```python
from build123d import *

# Parameters (mm, degrees)
RESSALTO_EXTRUS_O1_DEPTH                             = 4
FURO_DE_DI_METRO_6_0_6_1_D                           = 6
FURO_DE_DI_METRO_6_0_6_1_DEPTH                       = 2
FURO_DE_DI_METRO_6_0_6_1_TIP                         = 1.802581857
ESBO_O4_R                                            = 1.2
CORTE_EXTRUS_O1_DEPTH                                = 32.271167096
ESCAREADO_PARA_PARAFUSO_COM_CABE_A_ESCAR_D           = 3.4
ESCAREADO_PARA_PARAFUSO_COM_CABE_A_ESCAR_CSINK_D     = 6.3
ESCAREADO_PARA_PARAFUSO_COM_CABE_A_ESCAR_CSINK_ANGLE = 90
FILETE1_R                                            = 10
FILETE2_R                                            = 1


with BuildPart() as part:
    # Esboço1 → Ressalto-extrusão1 (new body)
    with BuildSketch(Plane(origin=(0, 0, 0), x_dir=(0, 0, -1), z_dir=(1, 0, 0))):
        with BuildLine():
            Line((0, 0), (0, 3.091839499))
            ThreePointArc((0, 3.091839499), (2.870368785, 6.92901728), (7.361966659, 5.259137398))
            Line((7.361966659, 5.259137398), (16.225984495, -7.134144996))
            Line((16.225984495, -7.134144996), (26, -16.908160501))
            Line((26, -16.908160501), (13, -16.908160501))
            Line((13, -16.908160501), (8, -11.908160501))
            Line((8, -11.908160501), (8, -8.399335203))
            Line((8, -8.399335203), (0, 0))
        make_face()
    extrude(amount=RESSALTO_EXTRUS_O1_DEPTH)

    # Furo de diâmetro Ø6.0 (6)1
    with Locations(Plane.ZY):
        with Locations((-4, 3.091839499)):
            Hole(FURO_DE_DI_METRO_6_0_6_1_D / 2, depth=FURO_DE_DI_METRO_6_0_6_1_DEPTH)
            with Locations((0, 0, -(FURO_DE_DI_METRO_6_0_6_1_DEPTH + FURO_DE_DI_METRO_6_0_6_1_TIP / 2))):  # 118° drill point
                Cone(0, FURO_DE_DI_METRO_6_0_6_1_D / 2, FURO_DE_DI_METRO_6_0_6_1_TIP, mode=Mode.SUBTRACT)

    # Esboço4 → Corte-extrusão1 (cut, through all)
    with BuildSketch(Plane(origin=(4, 0, 0), x_dir=(0, 0, -1), z_dir=(1, 0, 0))):
        with Locations((4, 3.091839499)):
            Circle(ESBO_O4_R)
    extrude(amount=-CORTE_EXTRUS_O1_DEPTH, mode=Mode.SUBTRACT)

    # Escareado para parafuso com cabeça escareada chata de M31 (through all)
    with Locations(Plane(origin=(4, 0, 0), x_dir=(0, 0, -1), z_dir=(1, 0, 0))):
        with Locations((15, -11.908160501)):
            CounterSinkHole(ESCAREADO_PARA_PARAFUSO_COM_CABE_A_ESCAR_D / 2, ESCAREADO_PARA_PARAFUSO_COM_CABE_A_ESCAR_CSINK_D / 2, counter_sink_angle=ESCAREADO_PARA_PARAFUSO_COM_CABE_A_ESCAR_CSINK_ANGLE)

    # Filete1
    # the kernel refuses this fillet: 10 mm, written as the material it adds along each edge
    with BuildSketch(Plane(origin=(0, -8.399335203, -8), x_dir=(0, 0.724110671276106, 0.6896837940274276), z_dir=(1, 0, 0))) as filete1_piece_1:
        with BuildLine():
            CenterArc((3.981744366, 10), FILETE1_R, 229.288374317, 40.711625683)
            Line((-2.540777842, 2.419979944), (-2.671228286, 2.268379543))
            ThreePointArc((-2.671228286, 2.268379543), (-1.40832568, 1.065167838), (-0.137936759, -0.144822134))
            Line((-0.137936759, -0.144822134), (0, -0.2))
            Line((0, -0.2), (3.981744366, -0.2))
            Line((3.981744366, -0.2), (3.981744366, 0))
        make_face()
    extrude(amount=4)
    with BuildSketch(Plane(origin=(0, -7.134144996, -16.225984495), x_dir=(0, -0.7071067811865512, -0.7071067811865437), z_dir=(1, 0, 0))) as filete1_piece_2:
        with BuildLine():
            CenterArc((FILETE1_R * 0.0824486959728, FILETE1_R), FILETE1_R, 260.573396821, 9.426603179)
            Line((-FILETE1_R * 0.0813353269941, FILETE1_R * 0.0135037791148), (-FILETE1_R * 0.0846110074534, -FILETE1_R * 0.00622614530291))
            Line((-FILETE1_R * 0.0846110074534, -FILETE1_R * 0.00622614530291), (-FILETE1_R * 0.00164897391946, -FILETE1_R * 0.02))
            Line((-FILETE1_R * 0.00164897391946, -FILETE1_R * 0.02), (FILETE1_R * 0.0824486959728, -FILETE1_R * 0.02))
            Line((FILETE1_R * 0.0824486959728, -FILETE1_R * 0.02), (FILETE1_R * 0.0824486959728, 0))
        make_face()
    extrude(amount=4)

    # Filete2
    filete2_edges = [part.edges().sort_by_distance(p)[0] for p in [
        (2, -16.908160501, -26),
    ]]
    fillet(filete2_edges, radius=FILETE2_R)


solid = part.part
```
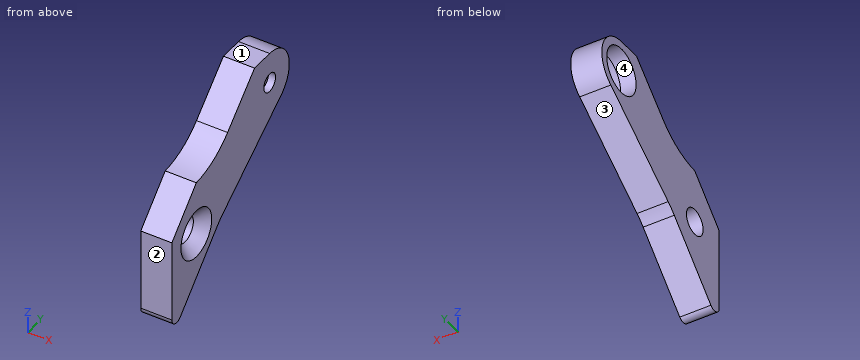
Build history of the part. All positions in model axes, mm. Face numbers are marked on the shaded views. Give positions to 0.01 mm unless a question says otherwise; leave off trailing zeros. Order: outer loops, then holes, each group sorted by start corner. A loop starts at its lowest first (then second) coordinate and runs counter-clockwise, first axis right, second up. Notation, with made-up numbers: M -10.75,21 L 15.25,21 A27 cw 15.25,52 Z; hole C 35.5,-11.75 d2. An arc over 180 degrees is marked long. Return JSON: item names as keys, results as strings.
Q1. Wall check: probe 1 along Z at (x, y) = (1.8, 5.5); probe 2 along Y at (x, z) = (3.75, -4); probe 3 along Y at (x, z) = (1.05, -4). Give the ranges that are in metal, low to high. Write a range as from..to.
Answer list:
{"probe 1": "z = -7.19..-5.79, -2.21..-0.81", "probe 2": "y = -4.2..1.89, 4.29..7.09", "probe 3": "y = -4.2..0.09, 6.09..7.09"}
Q2. Two-plate mould, pull along Y, no slides. Class the marked faces 1, 2, 3 and 4: pulls with the +Y half, pulls with the -Y half, needs draft (parallel to the pull), parting line crosses it, or undercut.
Answer list:
{"face 1": "needs draft", "face 2": "pulls with the -Y half", "face 3": "pulls with the +Y half", "face 4": "undercut"}
Q3. Flat gauge pin, fed straight in: pin 1 (3.5 mm diameter, centred on y = 3.09, z = -4, fed in from -X). Where does the tip first touch, or does it go through?
Answer list:
{"pin 1": "stops at x = 2.75"}
Q4. Band-saw the part on B-B (z = -4). Give the cut face in (x, y).
Answer list:
{"outline": "M 0,-4.2 L 4,-4.2 L 4,1.89 L 3.08,1.89 L 2,0.09 L 0,0.09 Z; M 0,6.09 L 2,6.09 L 3.08,4.29 L 4,4.29 L 4,7.09 L 0,7.09 Z"}
Q5. Band-saw the part on A-A (x = 1.3). Give the cut face in (y, z).
Answer list:
{"outline": "M -16.91,-23.59 A1 ccw -15.2,-24.29 L -7.72,-16.81 A10 cw -6.46,-15.75 L 5.26,-7.36 A4 ccw 3.09,0 L 0,0 L -5.52,-5.25 A10 cw -11.91,-8 L -16.91,-13 Z; hole C -11.91,-15 d3.4; hole C 3.09,-4 d6"}
Q6. Band-saw the part on C-C (x = 3.45). Give the cut face in (y, z).
Answer list:
{"outline": "M -16.91,-23.59 A1 ccw -15.2,-24.29 L -7.72,-16.81 A10 cw -6.46,-15.75 L 5.26,-7.36 A4 ccw 3.09,0 L 0,0 L -5.52,-5.25 A10 cw -11.91,-8 L -16.91,-13 Z; hole C -11.91,-15 d5.2; hole C 3.09,-4 d2.4"}
Q7. Band-saw the part on D-D (z = -15). Give the cut face in (x, y), then the cut area to 4 significant figures.
Answer list:
{"outline": "M 0,-16.91 L 4,-16.91 L 4,-15.06 L 2.55,-13.61 L 0,-13.61 Z; M 0,-10.21 L 2.55,-10.21 L 4,-8.76 L 4,-5.42 L 0,-5.42 Z", "area": "30.25 mm^2"}
